Input: part model. Units: mm. Frame: model coordinates. A direction names the side the tool comes from. Round coordinates to 2 decimals unless told otherwise and drop trailing zeros. Write each loop counter-clockwise with the first axis right and the second up, starting at its lowest first coordinate (ties: lowest second). Pieces come first, ordered by that corner, then holes. Notation, with made-up numbers: (-34, 44.25) - (3, 44.25) arc R24 cw to (3, 56.25) - close; hole circle Ø11 at (56.25, 77.5). An arc over 180 degrees is marked (long way). Use one line per item in the form item = value.
```python
from build123d import *

# Parameters (mm, degrees)
SKETCH_1_W                        = 240
SKETCH_1_H                        = 20
SM_BASE_FLANGE_1_DEPTH            = 2
SM_EDGE_FLANGE_1_STRIP_W          = 13.4732
SM_EDGE_FLANGE_1_STRIP_H          = 2
SM_EDGE_FLANGE_1_STRIP_CUT_DEPTH  = 20
SM_EDGE_FLANGE_1_RELIEF_W         = 14.4732
SM_EDGE_FLANGE_1_RELIEF_H         = 1
SM_EDGE_FLANGE_1_RELIEF_CUT_DEPTH = 2
SM_EDGE_FLANGE_1_DEPTH            = 20
SKETCH_10_R                       = 2.75
CUT_EXTRUDE_2_DEPTH               = 10
SKETCH_11_R                       = 2.75
SKETCH_11_R_2                     = 1.75
CUT_EXTRUDE_3_DEPTH               = 10


# Sheet-metal steps are written as plain solids
with BuildPart() as part:
    # Sketch 1 → 基体-法兰1 (new body)
    with BuildSketch(Plane.XY):
        with Locations((0, -10)):
            Rectangle(SKETCH_1_W, SKETCH_1_H)
    extrude(amount=-SM_BASE_FLANGE_1_DEPTH)

    # 边线-法兰1 strip (across the edge) → 边线-法兰1 strip cut (cut)
    with BuildSketch(Plane(origin=(-120, -20, 0), x_dir=(0, 1, 0), z_dir=(1, 0, 0))):
        with Locations((-2, -1)):
            Rectangle(SM_EDGE_FLANGE_1_STRIP_W, SM_EDGE_FLANGE_1_STRIP_H)
    sm_edge_flange_1_strip_cut = extrude(amount=SM_EDGE_FLANGE_1_STRIP_CUT_DEPTH, mode=Mode.SUBTRACT)

    # 边线-法兰1 relief (on the sheet) → 边线-法兰1 relief cut (cut)
    with BuildSketch(Plane(origin=(-120, -15.2634, 0), x_dir=(0, 1, 0), z_dir=(0, 0, 1))):
        with Locations((-6.2366, -20.5)):
            Rectangle(SM_EDGE_FLANGE_1_RELIEF_W, SM_EDGE_FLANGE_1_RELIEF_H)
    sm_edge_flange_1_relief_cut = extrude(amount=-SM_EDGE_FLANGE_1_RELIEF_CUT_DEPTH, mode=Mode.SUBTRACT)

    # 边线-法兰1 section (across the edge) → 边线-法兰1 (add)
    with BuildSketch(Plane(origin=(-120, -20, 0), x_dir=(0, 1, 0), z_dir=(1, 0, 0))):
        with BuildLine():
            Line((0, 2.7366), (0, 20))
            Line((0, 20), (2, 20))
            Line((2, 20), (2, 2.7366))
            ThreePointArc((2, 2.7366), (2.801531583, 0.801531583), (4.7366, 0))
            Line((4.7366, 0), (4.7366, -2))
            ThreePointArc((4.7366, -2), (1.38731802, -0.61268198), (0, 2.7366))
        make_face()
    sm_edge_flange_1 = extrude(amount=SM_EDGE_FLANGE_1_DEPTH)

    # 草图10 → 切除-拉伸2 (cut)
    with BuildSketch(Plane(origin=(0, -18, 0), x_dir=(1, 0, 0), z_dir=(0, 1, 0))):
        with Locations(Location((-110, -10, 0), (0, 0, 270))):
            Circle(SKETCH_10_R)
    cut_extrude_2 = extrude(amount=-CUT_EXTRUDE_2_DEPTH, mode=Mode.SUBTRACT)

    # 镜向1: 边线-法兰1 strip cut, 边线-法兰1 relief cut, 边线-法兰1, 切除-拉伸2 across plane
    add(sm_edge_flange_1_strip_cut.mirror(Plane(origin=(0, 0, 0), x_dir=(0, 0, 1), z_dir=(1, 0, 0))), mode=Mode.SUBTRACT)
    add(sm_edge_flange_1_relief_cut.mirror(Plane(origin=(0, 0, 0), x_dir=(0, 0, 1), z_dir=(1, 0, 0))), mode=Mode.SUBTRACT)
    add(sm_edge_flange_1.mirror(Plane(origin=(0, 0, 0), x_dir=(0, 0, 1), z_dir=(1, 0, 0))))
    add(cut_extrude_2.mirror(Plane(origin=(0, 0, 0), x_dir=(0, 0, 1), z_dir=(1, 0, 0))), mode=Mode.SUBTRACT)

    # 草图11 → 切除-拉伸3 (cut)
    with BuildSketch(Plane(origin=(0, 0, -2), x_dir=(-1, 0, 0), z_dir=(0, 0, -1))):
        with Locations((0, -10)):
            Circle(SKETCH_11_R)
        with Locations((-11, -10)):
            Circle(SKETCH_11_R)
        with Locations(Location((11, -10, 0), (0, 0, 180))):
            Circle(SKETCH_11_R)
        with Locations((-80, -10)):
            Circle(SKETCH_11_R_2)
        with Locations((-70, -10)):
            Circle(SKETCH_11_R_2)
        with Locations(Location((80, -10, 0), (0, 0, 180))):
            Circle(SKETCH_11_R_2)
        with Locations(Location((70, -10, 0), (0, 0, 180))):
            Circle(SKETCH_11_R_2)
    extrude(amount=-CUT_EXTRUDE_3_DEPTH, mode=Mode.SUBTRACT)


solid = part.part
```
(1) First-contact query: pin 1 Ø1 at (x, y) = (46.5, -8) entering from +Z; pin 2 Ø0.5 at (x, z) = (99.5, -1) entering from -Y; pin 3 Ø5 at (x, z) = (110, 10) entering from -Y; pin 4 Ø5 at (x, z) = (-109.5, 13) entering from +Y. Flat tips, straight axial feed; report the tip coordinate or a pass-through.
Derived:
pin_1 = 0
pin_2 = -14.26
pin_3 = through
pin_4 = -18
(2) Cut plane B-B on z = 4.75. Output: boundary loops of the cut face in (x, y).
Derived:
outline = (-120, -20) - (-100, -20) - (-100, -18) - (-120, -18) - close; (100, -20) - (120, -20) - (120, -18) - (100, -18) - close
(3) Draft query along X for faces 1 (the face through (120, -19, 6)), 2 (the face through (-112.685, -18.986, 9.404)), 3 (the face through (110, -20, 13)). Return one class per face: released by +X, released by -X, zero draft, split by the parting line, or undercut.
Derived:
face_1 = released by +X
face_2 = undercut
face_3 = zero draft
(4) Material intervals for L1, parallel to X at y = -19.4, z = 10; L2, parallel to Y at x = -80, z = -1.45; L3, parallel to Y at x = 11, z = -0.65, sorted ascending.
Derived:
L1 = -120 to -112.75, -107.25 to -100, 100 to 107.25, 112.75 to 120
L2 = -20 to -11.75, -8.25 to 0
L3 = -20 to -12.75, -7.25 to 0
(5) Cut plane D-D on x = -84.5. Output: boundary loops of the cut face in (y, z), then the cut area to 3 significant figures.
Derived:
outline = (-20, -2) - (0, -2) - (0, 0) - (-20, 0) - close
area = 40.0 mm^2
(6) Cut plane C-C on x = -110. Output: boundary loops of the cut face in (y, z).
Derived:
outline = (-20, 2.74) arc R4.74 ccw to (-15.26, -2) - (0, -2) - (0, 0) - (-15.26, 0) arc R2.74 cw to (-18, 2.74) - (-18, 7.25) - (-20, 7.25) - close; (-20, 12.75) - (-18, 12.75) - (-18, 20) - (-20, 20) - close
(7) Access query for faces 4 (the face through (110, -18, 13)), 5 (the face through (110.14, -18.576, -0.649)), 6 (the face through (-110.14, -18.576, -0.649)), 7 (the face through (100, -18.4, 6.7)), 8 (the face through (-1.7, -7.6, 0)). Directions: +Z, -Z, +X, -X, +Y, -Y. A direction counts if a zero-diameter tool reaches every point of the face in a straight line with its end or side. Return the directions, or none.
Derived:
face_4 = +Z, +X, -X, +Y
face_5 = -Z, +X, -Y
face_6 = -Z, -X, -Y
face_7 = +Z, -Z, -Y
face_8 = +Z, +Y
(8) Cut plane A-A on x = 0. Output: boundary loops of the cut face in (y, z).
Derived:
outline = (-20, -2) - (-12.75, -2) - (-12.75, 0) - (-20, 0) - close; (-7.25, -2) - (0, -2) - (0, 0) - (-7.25, 0) - close
